Verification items for the finished model (mm, model axes). A direction names the side the tool comes from. Round coordinates to 2 decimals unless told otherwise and drop trailing zeros. Write each loop counter-clockwise with the first axis right and the second up, starting at its lowest first coordinate (ties: lowest second). Pieces come first, ordered by that corner, then holes.
from build123d import *

# Parameters (mm, degrees)
ESQUISSE1_W                  = 16
ESQUISSE1_H                  = 14.5
ESQUISSE2_R                  = 4.1
ENL_V_MAT_EXTRU_1_DEPTH      = 4
CONG_2_R                     = 2
CONG_3_R                     = 2
ENL_V_START                  = 25
ESQUISSE3_R                  = 1.65
ENL_V_MAT_EXTRU_2_DEPTH      = 10
R_P_TITION_CIRCULAIRE1_COUNT = 8


with BuildPart() as part:
    # Esquisse1 → Révolution1 (revolve)
    with BuildSketch(Plane.XY, mode=Mode.PRIVATE) as r_volution1_sk:
        with Locations((8, 17.75)):
            Rectangle(ESQUISSE1_W, ESQUISSE1_H)
    revolve(r_volution1_sk.sketch.rotate(Axis((0, 0, 0), (1, 0, 0)), 90), axis=Axis((0, 0, 0), (1, 0, 0)))  # turned: the seam where the file's is

    # Esquisse2 → Enlèv. mat.-Extru.1 (cut)
    with BuildSketch(Plane.ZY):
        with BuildLine():
            Line((3.18, 14.761354951), (3.18, 18.999831578))
            ThreePointArc((3.18, 18.999831578), (0.08, 22.099831578), (-3.02, 18.999831578))
            Line((-3.02, 18.999831578), (-3.02, 14.794918046))
            ThreePointArc((-3.02, 14.794918046), (-7.479099439, 13.117662581), (-11.193708382, 10.13463826))
            Line((-11.193708382, 10.13463826), (-14.864336814, 12.253876573))
            ThreePointArc((-14.864336814, 12.253876573), (-19.099015566, 11.119197821), (-17.964336814, 6.88451907))
            Line((-17.964336814, 6.88451907), (-14.322774875, 4.782062304))
            ThreePointArc((-14.322774875, 4.782062304), (-15.099778753, 0.081741179), (-14.373708382, -4.626716692))
            Line((-14.373708382, -4.626716692), (-18.044336814, -6.745955005))
            ThreePointArc((-18.044336814, -6.745955005), (-19.179015566, -10.980633757), (-14.944336814, -12.115312509))
            Line((-14.944336814, -12.115312509), (-11.302774875, -10.012855743))
            ThreePointArc((-11.302774875, -10.012855743), (-7.620679314, -13.035921402), (-3.18, -14.761354951))
            Line((-3.18, -14.761354951), (-3.18, -18.999831578))
            ThreePointArc((-3.18, -18.999831578), (-0.08, -22.099831578), (3.02, -18.999831578))
            Line((3.02, -18.999831578), (3.02, -14.794918046))
            ThreePointArc((3.02, -14.794918046), (7.479099439, -13.117662581), (11.193708382, -10.13463826))
            Line((11.193708382, -10.13463826), (14.864336814, -12.253876573))
            ThreePointArc((14.864336814, -12.253876573), (19.099015566, -11.119197821), (17.964336814, -6.88451907))
            Line((17.964336814, -6.88451907), (14.322774875, -4.782062304))
            ThreePointArc((14.322774875, -4.782062304), (15.099778753, -0.081741179), (14.373708382, 4.626716692))
            Line((14.373708382, 4.626716692), (18.044336814, 6.745955005))
            ThreePointArc((18.044336814, 6.745955005), (19.179015566, 10.980633757), (14.944336814, 12.115312509))
            Line((14.944336814, 12.115312509), (11.302774875, 10.012855743))
            ThreePointArc((11.302774875, 10.012855743), (7.620679314, 13.035921402), (3.18, 14.761354951))
        make_face()
        Circle(ESQUISSE2_R, mode=Mode.SUBTRACT)
    extrude(amount=-ENL_V_MAT_EXTRU_1_DEPTH, mode=Mode.SUBTRACT)

    # Congé2
    cong_2_edges = [part.edges().sort_by_distance(p)[0] for p in [
        (4, 0, -10.5),
    ]]
    fillet(cong_2_edges, radius=CONG_2_R)

    # Congé3
    cong_3_edges = [part.edges().sort_by_distance(p)[0] for p in [
        (16, 0, -10.5),
    ]]
    fillet(cong_3_edges, radius=CONG_3_R)

    # Esquisse3 → Enlèv. mat.-Extru.2 (cut)
    with BuildSketch(Plane.XY.offset(ENL_V_START)):
        with Locations((12, 0)):
            Circle(ESQUISSE3_R)
    enl_v_mat_extru_2 = extrude(amount=-ENL_V_MAT_EXTRU_2_DEPTH, mode=Mode.SUBTRACT)

    # Répétition circulaire1: Enlèv. mat.-Extru.2 ×8 about axis
    r_p_tition_circulaire1_axis = Axis((0, 0, 0), (1, 0, 0))
    for i in range(1, R_P_TITION_CIRCULAIRE1_COUNT):
        add(enl_v_mat_extru_2.rotate(r_p_tition_circulaire1_axis, i * 360 / R_P_TITION_CIRCULAIRE1_COUNT), mode=Mode.SUBTRACT)


solid = part.part
Q1. Sectioned sample at D-D (y = 20). Enter the section's corners in (x, z), plus the area to 3 significant figures.
Recorded:
outline: (0, -15) - (16, -15) - (16, 15) - (0, 15) - (0, 3.01) - (4, 3.01) - (4, -2.85) - (0, -2.85) - close; hole circle Ø3.3 at (12, 0)
area: 448 mm2
Q2. Sectioned sample at B-B (z = 0). Enter the section's corners in (x, y), plus the area to 3 significant figures.
Recorded:
outline: (0, -25) - (10.35, -25) - (10.35, -15) - (13.65, -15) - (13.65, -25) - (16, -25) - (16, -12.5) arc R2 ccw to (14, -10.5) - (6, -10.5) arc R2 ccw to (4, -12.5) - (4, -22.1) - (0, -22.1) - close; (0, 22.1) - (4, 22.1) - (4, 12.5) arc R2 ccw to (6, 10.5) - (14, 10.5) arc R2 ccw to (16, 12.5) - (16, 25) - (13.65, 25) - (13.65, 15) - (10.35, 15) - (10.35, 25) - (0, 25) - close
area: 302 mm2
Q3. Release check for a two-part mould opening along Y. For faces 1 (the flat face through (0, 11, -11)), 2 (the flat face through (12, -15, 0)), 3 (the flat face through (11.977, -10.59, 10.623)) record: released by +Y, released by -Y, zero draft, split by the parting line, or undercut.
Recorded:
face 1: zero draft
face 2: released by -Y
face 3: undercut
Q4. Depth check by flat-ended pin: P1, Ø2, axis at x = 2.5, y = 16, coming from the +Z side; P2, Ø1.5, axis at y = -5.5, z = -13.5, coming from the -X side; P3, Ø2.5, axis at x = 12, z = 0, coming from the +Y side. Enter the tip coordinate at first touch or a pass-through.
Recorded:
P1: stops at z = 20
P2: stops at x = 4
P3: stops at y = 15
Q5. Tool access check on faces 4 (the flat face through (1.97, -11.08, -13.15)), 5 (the cylindrical face through (13.524, 20.07, 0.632)), 6 (the cylindrical face through (13.524, -0.632, 20.07)). Record the directions out of +Z, -Z, +X, -X, +Y, -Y that give a thin tool (end or side, any length) a straight path to the whole face; none if there is none.
Recorded:
face 4: -X
face 5: +Y
face 6: +Z
Q6. Sectioned sample at A-A (y = 0). Enter the section's corners in (x, z), plus the area to 3 significant figures.
Recorded:
outline: (0, -25) - (10.35, -25) - (10.35, -15) - (13.65, -15) - (13.65, -25) - (16, -25) - (16, -12.5) arc R2 ccw to (14, -10.5) - (6, -10.5) arc R2 ccw to (4, -12.5) - (4, -15.1) - (0, -15.1) - close; (0, 15.1) - (4, 15.1) - (4, 12.5) arc R2 ccw to (6, 10.5) - (14, 10.5) arc R2 ccw to (16, 12.5) - (16, 25) - (13.65, 25) - (13.65, 15) - (10.35, 15) - (10.35, 25) - (0, 25) - close
area: 358 mm2
Q7. Material ranges on line 1 along X through (y, z) = (23, 0); line 2 along Y through (x, z) = (11.25, -0.5); line 3 along X through (y, z) = (17.5, 0), recorded low to high.
Recorded:
line 1: x = 0 to 10.35, 13.65 to 16
line 2: y = -15 to -10.49, 10.49 to 15
line 3: x = 4 to 10.35, 13.65 to 16
